```python
from build123d import *

# Parameters (mm, degrees)
SKETCH1_R           = 1.5
BOSS_EXTRUDE1_DEPTH = 0.5


with BuildPart() as part:
    # Sketch1 → Boss-Extrude1 (new body)
    with BuildSketch(Plane(origin=(0, 0, 0), x_dir=(1, 0, 0), z_dir=(0, 1, 0))):
        Polygon((-6.55, -7.183333333), (-7.5, -7.5), (-7.5, -12.5), (7.5, -12.5), (7.5, -2.5), (6.55, -2.816666667), (6.45, -2.85), (5.55, -3.15), (5.45, -3.183333333), (4.55, -3.483333333), (4.45, -3.516666667), (3.55, -3.816666667), (3.45, -3.85), (2.55, -4.15), (2.45, -4.183333333), (1.55, -4.483333333), (1.45, -4.516666667), (0.55, -4.816666667), (0.45, -4.85), (-0.45, -5.15), (-0.55, -5.183333333), (-1.45, -5.483333333), (-1.55, -5.516666667), (-2.45, -5.816666667), (-2.55, -5.85), (-3.45, -6.15), (-3.55, -6.183333333), (-4.45, -6.483333333), (-4.55, -6.516666667), (-5.45, -6.816666667), (-5.55, -6.85), (-6.45, -7.15), align=None)
        with Locations((-3.75, -10)):
            Circle(SKETCH1_R, mode=Mode.SUBTRACT)
        with Locations((3.75, -10)):
            Circle(SKETCH1_R, mode=Mode.SUBTRACT)
        Polygon((6.55, -2.816666667), (7.5, -2.5), (7.5, 12.5), (6.55, 12.5), align=None)
        Polygon((5.55, -3.15), (6.45, -2.85), (6.45, 12.5), (5.55, 12.5), align=None)
        Polygon((4.55, -3.483333333), (5.45, -3.183333333), (5.45, 12.5), (4.55, 12.5), align=None)
        Polygon((3.55, -3.816666667), (4.45, -3.516666667), (4.45, 12.5), (3.55, 12.5), align=None)
        Polygon((2.55, -4.15), (3.45, -3.85), (3.45, 12.5), (2.55, 12.5), align=None)
        Polygon((1.55, -4.483333333), (2.45, -4.183333333), (2.45, 12.5), (1.55, 12.5), align=None)
        Polygon((0.55, -4.816666667), (1.45, -4.516666667), (1.45, 12.5), (0.55, 12.5), align=None)
        Polygon((-0.45, 12.5), (-0.45, -5.15), (0.45, -4.85), (0.45, 12.5), align=None)
        Polygon((-1.45, 12.5), (-1.45, -5.483333333), (-0.55, -5.183333333), (-0.55, 12.5), align=None)
        Polygon((-2.45, 12.5), (-2.45, -5.816666667), (-1.55, -5.516666667), (-1.55, 12.5), align=None)
        Polygon((-3.45, 12.5), (-3.45, -6.15), (-2.55, -5.85), (-2.55, 12.5), align=None)
        Polygon((-4.45, 12.5), (-4.45, -6.483333333), (-3.55, -6.183333333), (-3.55, 12.5), align=None)
        Polygon((-5.45, 12.5), (-5.45, -6.816666667), (-4.55, -6.516666667), (-4.55, 12.5), align=None)
        Polygon((-6.45, 12.5), (-6.45, -7.15), (-5.55, -6.85), (-5.55, 12.5), align=None)
        Polygon((-7.5, 12.5), (-7.5, -7.5), (-6.55, -7.183333333), (-6.55, 12.5), align=None)
    extrude(amount=BOSS_EXTRUDE1_DEPTH)


solid = part.part
```
Geometry: final body of the model. Coordinates: model frame, mm. Give positions to 0.01 mm unless a question says otherwise; leave off trailing zeros. Order: outer loops, then holes, each group sorted by start corner. A loop starts at its lowest first (then second) coordinate and runs counter-clockwise, first axis right, second up. Notation, with made-up numbers: (-32, 76) -> (-10, 76) arc R6 ccw to (-10, 85) -> close; hole circle Ø3 at (17, -35). An arc over 180 degrees is marked (long way). Write each question's results on one line, items separated by ' | '. Start each with the question number.
1) Line query: line 1 (X direction, y = 0.2, z = 10); line 2 (Z direction, x = -3.75, y = 0.3); line 3 (Z direction, x = -3.5, y = 0.4). Output: solid intervals per line, ascending. Write a range as from..to.
2) Section B-B (x = 4). Return loops of the section in (y, z).
3) Draft query along Z for faces 1 (the flat face through (0, 0.5, 0)), 2 (the cylindrical face through (5.136, 0.246, 10.575)). Return one class per face: pulls with the +Z half, pulls with the -Z half, needs draft (parallel to the pull), parting line crosses it, or undercut.
4) Section C-C (z = -7.5). Count the separate pieces of the cut face and the enclosed holes in it, then the cut area to 3 significant figures.
5) First-contact query: pin 1 (4 mm diameter, centred on x = 3.75, z = 10, fed in from -Y). Flat tip, straight axial feed; report the tip coordinate or a pass-through.
6) Section A-A (z = 10). Return loops of the section in (x, y).
Calculated:
1) line 1: -7.5..-5.25, -2.25..2.25, 5.25..7.5 | line 2: -12.5..8.5, 11.5..12.5 | line 3: 6.17..8.52, 11.48..12.5
2) outline: (0, -12.5) -> (0.5, -12.5) -> (0.5, 8.52) -> (0, 8.52) -> close; (0, 11.48) -> (0.5, 11.48) -> (0.5, 12.5) -> (0, 12.5) -> close
3) face 1: needs draft | face 2: undercut
4) separate pieces: 15 | enclosed holes: 0 | area: 6.80 mm2
5) pin 1: y = 0
6) outline: (-7.5, 0) -> (-5.25, 0) -> (-5.25, 0.5) -> (-7.5, 0.5) -> close; (-2.25, 0) -> (2.25, 0) -> (2.25, 0.5) -> (-2.25, 0.5) -> close; (5.25, 0) -> (7.5, 0) -> (7.5, 0.5) -> (5.25, 0.5) -> close
